```python
from build123d import *

# Parameters (mm, degrees)
F0_R     = 3.96875
F1_DEPTH = 6.746875
F2_R     = 3.175
F3_DEPTH = 50.8


with BuildPart() as f1:
    # F0 (on Top) → F1 (new body)
    with BuildSketch(Plane.XY):
        Polygon((3.666174, 6.35), (-3.666174, 6.35), (-7.332348, 0), (-3.666174, -6.35), (3.666174, -6.35), (7.332348, 0), align=None)
        Circle(F0_R, mode=Mode.SUBTRACT)
    extrude(amount=F1_DEPTH)

    # F2 (on face) → F3 (join)
    with BuildSketch(Plane(origin=(0, 6.35, 0), x_dir=(-1, 0, 0), z_dir=(0, 1, 0))):
        with Locations((0, 3.373438)):
            Circle(F2_R)
    extrude(amount=F3_DEPTH)


solid = f1.part
```
Input: part model. Units: mm. Frame: model coordinates. A direction names the side the tool comes from. Give positions to 0.01 mm unless a question says otherwise; leave off trailing zeros. Order: outer loops, then holes, each group sorted by start corner. A loop starts at its lowest first (then second) coordinate and runs counter-clockwise, first axis right, second up. Notation, with made-up numbers: (40.5, 54.25) - (59.5, 54.25) arc R13 ccw to (59.5, 74.25) - close; hole circle Ø10 at (38, 67). An arc over 180 degrees is marked (long way). Use a Markdown table: item, result.
(1) Draft query along Y for faces 3 (the cylindrical face through (0.688, 31.394, 0.274)), 4 (the flat face through (-5.474, 3.219, 3.326)), 5 (the cylindrical face through (-0.86, -3.874, 3.326)). Return one class per face: released by +Y, released by -Y, zero draft, split by the parting line, or undercut.
Computed values:
| item | result |
|---|---|
| face 3 | zero draft |
| face 4 | released by +Y |
| face 5 | undercut |
(2) Access query for faces 1 (the flat face through (0, -6.35, 3)), 2 (the flat face through (2.5, 6.35, 1.1)). Directions: +Z, -Z, +X, -X, +Y, -Y. A direction counts if a zero-diameter tool reaches every point of the face in a straight line with its end or side. Return the directions, or none.
Computed values:
| item | result |
|---|---|
| face 1 | +Z, -Z, +X, -X, -Y |
| face 2 | +Y |
(3) Section query A-A (x = 0). Output: boundary loops of the cut face in (y, z).
Computed values:
| item | result |
|---|---|
| outline | (-6.35, 0) - (-3.97, 0) - (-3.97, 6.75) - (-6.35, 6.75) - close; (3.97, 0) - (6.35, 0) - (6.35, 0.2) - (57.15, 0.2) - (57.15, 6.55) - (6.35, 6.55) - (6.35, 6.75) - (3.97, 6.75) - close |
(4) Section query C-C (z = 1). Output: boundary loops of the cut face in (x, y), then the cut area to 3 significant figures.
Computed values:
| item | result |
|---|---|
| outline | (-7.33, 0) - (-3.67, -6.35) - (3.67, -6.35) - (7.33, 0) - (3.67, 6.35) - (2.11, 6.35) - (2.11, 57.15) - (-2.11, 57.15) - (-2.11, 6.35) - (-3.67, 6.35) - close; hole circle Ø7.94 at (0, 0) |
| area | 304 mm2 |
(5) Pin query (flat end, axial travel): pin 1 (3 mm diameter, centred on y = 23, z = 4.5, fed in from +X) (3 decimals); pin 2 (2 mm diameter, centred on y = 13, z = 5.5, fed in from -X); pin 3 (6 mm diameter, centred on x = 2.5, y = 22.5, fed in from +Z); pin 4 (5 mm diameter, centred on x = 0, y = 0, fed in from +Z). Return the tip coordinate at first contact, or that it passes through.
Computed values:
| item | result |
|---|---|
| pin 1 | stops at x = 3.175 |
| pin 2 | stops at x = -2.97 |
| pin 3 | stops at z = 6.55 |
| pin 4 | passes through |
(6) Section query D-D (x = 2.5). Output: boundary loops of the cut face in (y, z), then the cut area to 3 significant figures.
Computed values:
| item | result |
|---|---|
| outline | (-6.35, 0) - (-3.08, 0) - (-3.08, 6.75) - (-6.35, 6.75) - close; (3.08, 0) - (6.35, 0) - (6.35, 1.42) - (57.15, 1.42) - (57.15, 5.33) - (6.35, 5.33) - (6.35, 6.75) - (3.08, 6.75) - close |
| area | 243 mm2 |
(7) Line query: line 1 (Y direction, x = 0, z = 3.75); line 2 (Z direction, x = 0, y = 15); line 3 (Y direction, x = -0.5, z = 4). Output: solid intervals per line, ascending. Write a range as from..to.
Computed values:
| item | result |
|---|---|
| line 1 | y = -6.35..-3.97, 3.97..57.15 |
| line 2 | z = 0.2..6.55 |
| line 3 | y = -6.35..-3.94, 3.94..57.15 |
(8) Section query B-B (y = 2). Output: boundary loops of the cut face in (x, z).
Computed values:
| item | result |
|---|---|
| outline | (-6.18, 0) - (-3.43, 0) - (-3.43, 6.75) - (-6.18, 6.75) - close; (3.43, 0) - (6.18, 0) - (6.18, 6.75) - (3.43, 6.75) - close |
